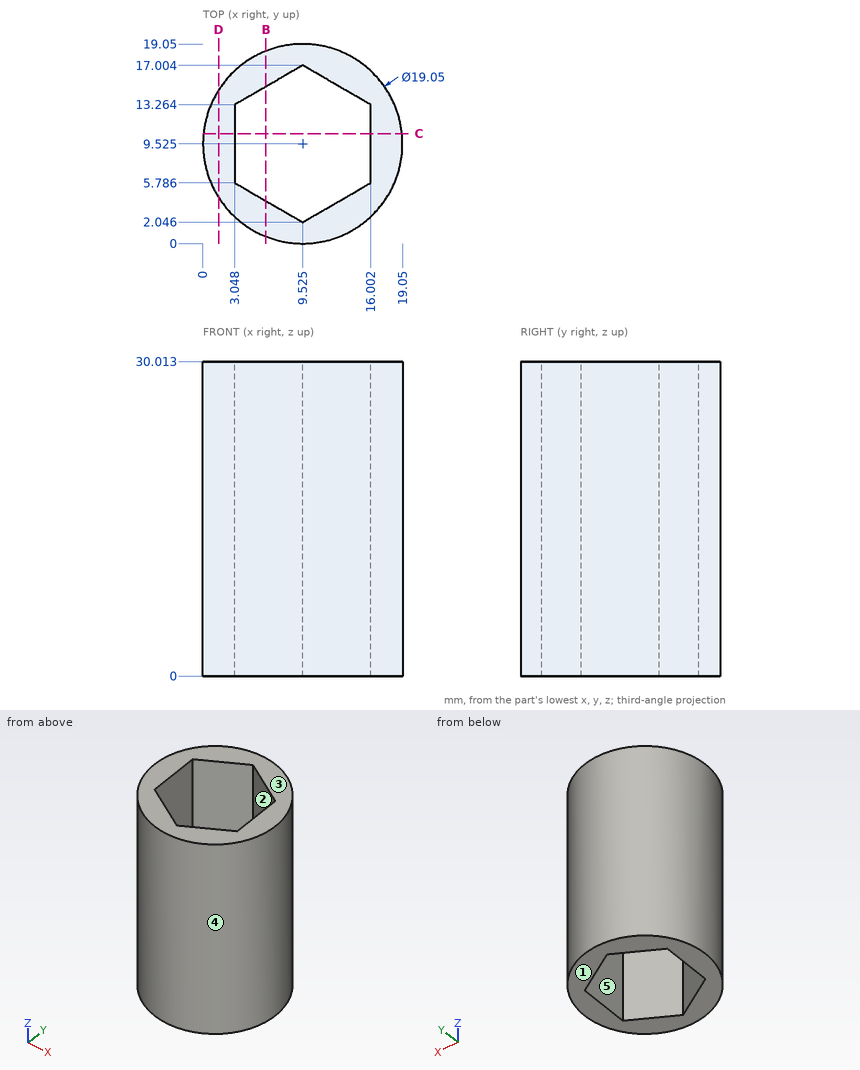
Design review of the part shown in the three views and the two pictorial views. Dimensions are in mm from the part's minimum x, y and z. A direction names the side the tool comes from. Round coordinates to 2 decimals unless told otherwise and drop trailing zeros. Write each loop counter-clockwise with the first axis right and the second up, starting at its lowest first coordinate (ties: lowest second). Pieces come first, ordered by that corner, then holes. Notation, with made-up numbers: (41, 84) -> (80, 84) arc R8 cw to (80, 90) -> close; hole circle Ø10 at (85.5, 75). An arc over 180 degrees is marked (long way). Use one line per item in the form item = value.
1) Take a section at D-D, the plane x = 1.5. Write out the cut boundary in (y, z) (1 decimal), and give its area (3 significant figures).
Found:
outline = (4.4, 0) -> (14.7, 0) -> (14.7, 30) -> (4.4, 30) -> close
area = 308 mm2
2) Clearance check with flat-ended pins moving along their axes: pin 1 (6 mm diameter, centred on x = 13, z = 18, fed in from -Y); pin 2 (1.5 mm diameter, centred on y = 15.5, z = 11, fed in from -X); pin 3 (1 mm diameter, centred on x = 10, y = 5, fed in from -Z); pin 4 (1 mm diameter, centred on x = 14.5, z = 22, fed in from -Y). State where each tip first meets the part, or that it passes through.
Found:
pin_1 = 0.01
pin_2 = 1.56
pin_3 = through
pin_4 = 1.12
3) Tool access review of the marked faces 1 and 2: name each direction out of +Z, -Z, +X, -X, +Y, -Y from which nothing blocks a thin tool from reaching the whole face with its end or side.
Found:
face_1 = -Z, +X, -X, +Y, -Y
face_2 = +Z, -Z
4) To check wall thickness, follow L1, parallel to X at y = 14.25, z = 29 (1 decimal); L2, parallel to X at y = 11.25, z = 18; L3, parallel to Y at x = 11.25, z = 1.5. State the ranges of each line that lie inside material, in increasing order. Write a range as from..to.
Found:
L1 = 1.3..4.8, 14.3..17.8
L2 = 0.16..3.05, 16..18.89
L3 = 0.16..3.04, 16.01..18.89
5) Take a section at C-C, the plane y = 10.5. Write out the cut boundary in (x, z), and give its area (3 significant figures).
Found:
outline = (0.05, 0) -> (3.05, 0) -> (3.05, 30.01) -> (0.05, 30.01) -> close; (16, 0) -> (19, 0) -> (19, 30.01) -> (16, 30.01) -> close
area = 180 mm2
6) Take a section at B-B, the plane x = 6. Write out the cut boundary in (y, z).
Found:
outline = (0.68, 0) -> (4.08, 0) -> (4.08, 30.01) -> (0.68, 30.01) -> close; (14.97, 0) -> (18.37, 0) -> (18.37, 30.01) -> (14.97, 30.01) -> close
7) Mouldability with a two-part tool opening along X and no side actions: class the marked faces 3, 4 and 5 as +X half, -X half, draft (parallel to the pull), parting line (faces both ways), or undercut.
Found:
face_3 = draft
face_4 = parting line
face_5 = undercut
